Design review of the part built by this model. Coordinates are the model's own, in mm. Round coordinates to 2 decimals unless told otherwise and drop trailing zeros. Write each loop counter-clockwise with the first axis right and the second up, starting at its lowest first coordinate (ties: lowest second). Pieces come first, ordered by that corner, then holes. Notation, with made-up numbers: (48.5, -40) - (84.5, -40) arc R11 ccw to (84.5, -31) - close; hole circle Ø3 at (86, -8.5). An arc over 180 degrees is marked (long way). Use one line per item in the form item = value.
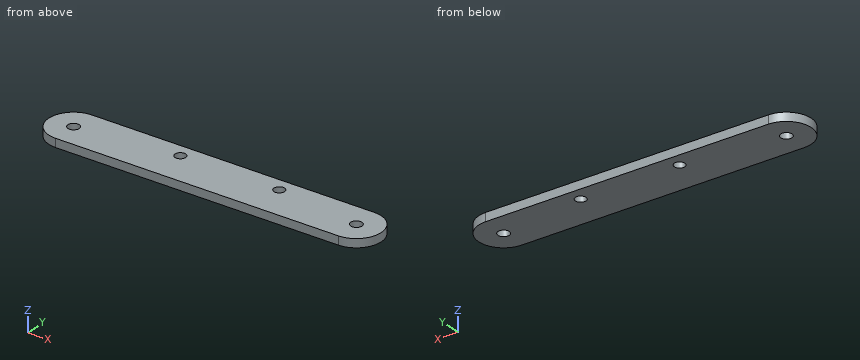
```python
from build123d import *

# Parameters (mm, degrees)
ESQUISSE1_R             = 4
BOSS_EXTRU_1_DEPTH      = 6
ENL_V_MAT_EXTRU_1_REACH = 134.912
ESQUISSE2_R             = 3.75


with BuildPart() as part:
    # Esquisse1 → Boss.-Extru.1 (new body)
    with BuildSketch(Plane.XY):
        with BuildLine():
            Line((-114.118449195, 17.5), (85.881550805, 17.5))
            ThreePointArc((85.881550805, 17.5), (103.381550805, 0), (85.881550805, -17.5))
            Line((85.881550805, -17.5), (-114.118449195, -17.5))
            ThreePointArc((-114.118449195, -17.5), (-131.618449195, 0), (-114.118449195, 17.5))
        make_face()
        with Locations((-114.118449195, 0)):
            Circle(ESQUISSE1_R, mode=Mode.SUBTRACT)
        with Locations((85.881550805, 0)):
            Circle(ESQUISSE1_R, mode=Mode.SUBTRACT)
    extrude(amount=BOSS_EXTRU_1_DEPTH)

    # Esquisse2 → Enlèv. mat.-Extru.1 (cut, up to next)
    with BuildSketch(Plane.XY.offset(6), mode=Mode.PRIVATE) as enl_v_mat_extru_1_sk1:
        with Locations((-44.118449195, 7.5)):
            Circle(ESQUISSE2_R)
    enl_v_mat_extru_1_tool1 = extrude(enl_v_mat_extru_1_sk1.sketch, amount=-ENL_V_MAT_EXTRU_1_REACH, mode=Mode.PRIVATE) & part.part
    # Esquisse2 → Enlèv. mat.-Extru.1 (cut, up to next)
    with BuildSketch(Plane.XY.offset(6), mode=Mode.PRIVATE) as enl_v_mat_extru_1_sk2:
        with Locations((25.881550805, 7.5)):
            Circle(ESQUISSE2_R)
    enl_v_mat_extru_1_tool2 = extrude(enl_v_mat_extru_1_sk2.sketch, amount=-ENL_V_MAT_EXTRU_1_REACH, mode=Mode.PRIVATE) & part.part
    add(enl_v_mat_extru_1_tool1.solids().sort_by_distance((-44.118449, 7.5, 6))[0], mode=Mode.SUBTRACT)
    add(enl_v_mat_extru_1_tool2.solids().sort_by_distance((25.881551, 7.5, 6))[0], mode=Mode.SUBTRACT)


solid = part.part
```
Q1. We need section C-C on y = -10.5. Write out the cut boundary in (x, z), then the cut area to 3 significant figures.
Calculated:
outline = (-128.12, 0) - (99.88, 0) - (99.88, 6) - (-128.12, 6) - close
area = 1,370 mm2
Q2. We need section A-A on y = 0. Write out the cut boundary in (x, z), then the cut area to 3 significant figures.
Calculated:
outline = (-131.62, 0) - (-118.12, 0) - (-118.12, 6) - (-131.62, 6) - close; (-110.12, 0) - (81.88, 0) - (81.88, 6) - (-110.12, 6) - close; (89.88, 0) - (103.38, 0) - (103.38, 6) - (89.88, 6) - close
area = 1,310 mm2
Q3. To check wall thickness, follow line 1 along X through (y, z) = (8.5, 1.55); line 2 along X through (y, z) = (7, 0.3); line 3 along Y through (x, z) = (-113, 1.75). State the ranges of each line that lie inside material, in increasing order. Write a range as from..to.
Calculated:
line_1 = -129.42..-47.73, -40.5..22.27, 29.5..101.18
line_2 = -130.16..-47.83, -40.4..22.17, 29.6..101.92
line_3 = -17.5..-3.84, 3.84..17.5
Q4. We need section D-D on y = 14.5. Write out the cut boundary in (x, z), then the cut area to 3 significant figures.
Calculated:
outline = (-123.92, 0) - (95.68, 0) - (95.68, 6) - (-123.92, 6) - close
area = 1,320 mm2
Q5. We need section B-B on z = 4.75. Write out the cut boundary in (x, y).
Calculated:
outline = (-114.12, -17.5) - (85.88, -17.5) arc R17.5 ccw to (85.88, 17.5) - (-114.12, 17.5) arc R17.5 ccw to start; hole circle Ø8 at (-114.12, 0); hole circle Ø7.5 at (-44.12, 7.5); hole circle Ø7.5 at (25.88, 7.5); hole circle Ø8 at (85.88, 0)
Q6. For P1, Ø5, axis at x = -114.12, y = 0, coming from the -Z side; P2, Ø2, axis at y = -5, z = 4.5, coming from the +X side, all flat-tipped, find the tip position at first contact; note any pin that passes through.
Calculated:
P1 = through
P2 = 102.92
